Read the model definition and answer for the solid it produces. Units are mm, in the model's axes. A direction names the side the tool comes from. Round coordinates to 2 decimals unless told otherwise and drop trailing zeros. Write each loop counter-clockwise with the first axis right and the second up, starting at its lowest first coordinate (ties: lowest second). Pieces come first, ordered by that corner, then holes. Notation, with made-up numbers: (-6, 70) - (20, 70) arc R28 ccw to (20, 88) - close; hole circle Ø5 at (75, 77.5). An arc over 180 degrees is marked (long way). Answer as CSV lines item,"result". Start each with the question number.
1) Find section B-B on z = 0.45. Determine the outline of the cut face in (x, y), then the cut area to 3 significant figures.
2) Find section A-A on y = -5.5. Determine the outline of the cut face in (x, z), then the cut area to 3 significant figures.
3) Find section D-D on y = 6.25. Determine the outline of the cut face in (x, z), then the cut area to 3 significant figures.
4) For a pull along Y with two mould halves and no side action, classify faces 5 (the flat face through (0, 11.1, 1)), 6 (the flat face through (-0.2, -11.1, 0.4)), 7 (the flat face through (0, -6, 1.42)) as +Y half, -Y half, draft (parallel to the pull), parting line (faces both ways), or undercut.
5) Find section C-C on x = 11. Determine the outline of the cut face in (y, z).
6) Which of the six approach directions +Z, -Z, +X, -X, +Y, -Y give full straight-line access (tool end or side, diameter ignored) to faces 1 (the flat face through (0, 3, 1.52)), 2 (the flat face through (-0.2, -6.8, 0.82)), 3 (the flat face through (0, 0, 0)), 4 (the flat face through (0, -9, 0.92))?
7) Consider line 1 along Z through (x, y) = (9.75, 2); line 2 along Y through (x, z) = (-9.75, 1.2); line 3 along Y through (x, z) = (-5.5, 0.7). Determine where each line is inside the solid, lowest interval first.
8) Each of these flat-tipped pins is pushed along its axis until it touches: pin 1 (0.7 mm diameter, centred on x = 1, z = 1, fed in from -Y); pin 2 (4.5 mm diameter, centred on x = 1, y = -9, fed in from +Z); pin 3 (1 mm diameter, centred on y = -12, z = -0.5, fed in from -X). Where does it stop, or does it pass through?
from build123d import *

# Parameters (mm, degrees)
SKETCH_W     = 25.9
SKETCH_H     = 22.2
PAD_DEPTH    = 0.82
SKETCH001_W  = 25.9
SKETCH001_H  = 17.65
PAD001_DEPTH = 0.6
SKETCH002_W  = 24.7
SKETCH002_H  = 15.42
PAD002_DEPTH = 0.1
PAD003_DEPTH = 0.1
PAD004_DEPTH = 7
PAD005_DEPTH = 0.1


with BuildPart() as part:
    # Sketch → Pad (new body)
    with BuildSketch(Plane.XY):
        Rectangle(SKETCH_W, SKETCH_H)
    extrude(amount=PAD_DEPTH)

    # Sketch001 (on Face6 of Pad) → Pad001 (join)
    with BuildSketch(Plane.XY.offset(0.82)):
        with Locations((0, 2.275)):
            Rectangle(SKETCH001_W, SKETCH001_H)
    extrude(amount=PAD001_DEPTH)

    # Sketch002 (on Face10 of Pad001) → Pad002 (join)
    with BuildSketch(Plane.XY.offset(1.42)):
        with Locations((0, 2.79)):
            Rectangle(SKETCH002_W, SKETCH002_H)
    extrude(amount=PAD002_DEPTH)

    # Sketch003 (on Face7 of Pad002) → Pad003 (join)
    with BuildSketch(Plane.XY.offset(0.82)):
        with BuildLine():
            Line((-7.1, -7), (7.1, -7))
            ThreePointArc((7.5, -7.4), (7.382843, -7.117157), (7.1, -7))
            Line((7.5, -7.4), (7.5, -10.4))
            ThreePointArc((7.1, -10.8), (7.382843, -10.682843), (7.5, -10.4))
            Line((7.1, -10.8), (7, -10.8))
            Line((7, -10.8), (7, -11.1))
            Line((7, -11.1), (-7, -11.1))
            Line((-7, -11.1), (-7, -10.8))
            Line((-7, -10.8), (-7.1, -10.8))
            ThreePointArc((-7.5, -10.4), (-7.382843, -10.682843), (-7.1, -10.8))
            Line((-7.5, -10.4), (-7.5, -7.4))
            ThreePointArc((-7.1, -7), (-7.382843, -7.117157), (-7.5, -7.4))
        make_face()
    extrude(amount=PAD003_DEPTH)

    # Sketch004 → Pad004 (join, symmetric)
    with BuildSketch(Plane.YZ):
        with BuildLine():
            ThreePointArc((-11.1, 0.82), (-12.01, -0.09), (-11.1, -1))
            Line((-11.1, -1), (-4.18, -1))
            Line((-4.18, -1), (-4.18, -1.1))
            Line((-11.1, -1.1), (-4.18, -1.1))
            ThreePointArc((-11.1, 0.92), (-12.11, -0.09), (-11.1, -1.1))
            Line((-11.1, 0.82), (-11.1, 0.92))
        make_face()
    extrude(amount=PAD004_DEPTH, both=True)

    # Sketch005 (on Face34 of Pad004) → Pad005 (join)
    with BuildSketch(Plane(origin=(0, 0, -1.1), x_dir=(1, 0, 0), z_dir=(0, 0, -1))):
        with BuildLine():
            Line((-9, 4.2), (9, 4.2))
            Line((9, 4.2), (9, 8.9))
            ThreePointArc((9, 8.9), (8.42, 10.35), (7, 11))
            Line((7, 11), (-7, 11))
            ThreePointArc((-7, 11), (-8.42, 10.35), (-9, 8.9))
            Line((-9, 8.9), (-9, 4.2))
        make_face()
    extrude(amount=-PAD005_DEPTH)


solid = part.part
Check values:
1,outline,"(-12.95, -11.1) - (12.95, -11.1) - (12.95, 11.1) - (-12.95, 11.1) - close; (-7, -11.95) - (7, -11.95) - (7, -11.83) - (-7, -11.83) - close"
1,area,"577 mm^2"
2,outline,"(-12.95, 0) - (12.95, 0) - (12.95, 1.42) - (-12.95, 1.42) - close; (-9, -1.1) - (9, -1.1) - (9, -1) - (-9, -1) - close"
2,area,"38.6 mm^2"
3,outline,"(-12.95, 0) - (12.95, 0) - (12.95, 1.42) - (12.35, 1.42) - (12.35, 1.52) - (-12.35, 1.52) - (-12.35, 1.42) - (-12.95, 1.42) - close"
3,area,"39.2 mm^2"
4,face 5,"+Y half"
4,face 6,"undercut"
4,face 7,"draft"
5,outline,"(-11.1, 0) - (11.1, 0) - (11.1, 1.42) - (10.5, 1.42) - (10.5, 1.52) - (-4.92, 1.52) - (-4.92, 1.42) - (-6.55, 1.42) - (-6.55, 0.82) - (-11.1, 0.82) - close"
6,face 1,"+Z, +X, -X, +Y, -Y"
6,face 2,"+Z"
6,face 3,"+X, -X, +Y"
6,face 4,"+Z, +X, -X, -Y"
7,line 1,"z = 0 to 1.52"
7,line 2,"y = -6.55 to 11.1"
7,line 3,"y = -11.73 to -11.55, -11.1 to 11.1"
8,pin 1,"stops at y = -11.79"
8,pin 2,"stops at z = 0.92"
8,pin 3,"stops at x = -7"
